```python
from build123d import *

# Parameters (mm, degrees)
SKETCH1_W           = 100
SKETCH1_H           = 275
BOSS_EXTRUDE1_DEPTH = 10
SKETCH2_W           = 60
SKETCH2_H           = 5
BOSS_EXTRUDE2_DEPTH = 5
SKETCH3_R           = 10
CUT_EXTRUDE1_DEPTH  = 152.348108677


with BuildPart() as part:
    # Sketch1 → Boss-Extrude1 (new body)
    with BuildSketch(Plane.XY):
        Rectangle(SKETCH1_W, SKETCH1_H)
    extrude(amount=BOSS_EXTRUDE1_DEPTH)

    # Sketch2 → Boss-Extrude2 (add)
    with BuildSketch(Plane(origin=(0, 137.5, 0), x_dir=(1, 0, 0), z_dir=(0, 1, 0))):
        with Locations((0, -5)):
            Rectangle(SKETCH2_W, SKETCH2_H)
    extrude(amount=BOSS_EXTRUDE2_DEPTH)

    # Sketch3 → Cut-Extrude1 (cut, through all)
    with BuildSketch(Plane.XY.offset(10)):
        with Locations((25, -117.5)):
            Circle(SKETCH3_R)
        with Locations(Location((-25, -117.5, 0), (0, 0, 180))):
            Circle(SKETCH3_R)
    extrude(amount=-CUT_EXTRUDE1_DEPTH, mode=Mode.SUBTRACT)


solid = part.part
```
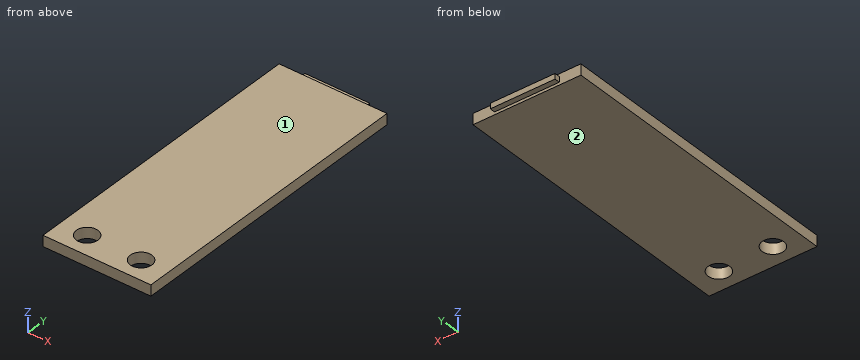
Read the model definition and answer for the solid it produces. Units are mm, in the model's axes. Face numbers are marked on the shaded views. Give positions to 0.01 mm unless a question says otherwise; leave off trailing zeros. Write each loop counter-clockwise with the first axis right and the second up, starting at its lowest first coordinate (ties: lowest second). Pieces come first, ordered by that corner, then holes. Notation, with made-up numbers: (66, -22.75) - (116, -22.75) arc R12 ccw to (116, -11.75) - close; hole circle Ø8 at (-35, -11.75). An arc over 180 degrees is marked (long way). Write item = value, one per line. Start each with the question number.
Item 1: Find section A-A (y = -117.5). Give the vertices of the cut face in (x, z).
Item 2: Find section C-C (z = 4.25). Give the vertices of the cut face in (x, y).
Item 3: The mould has two halves that part along Z. Classify the marked faces 1 and 2: +Z half, -Z half, draft (parallel to the pull), parting line (faces both ways), or undercut.
Item 4: Find section B-B (x = -25). Give the vertices of the cut face in (y, z), then the cut area to 4 significant figures.
Item 5: Find the intervals of material crossed by probe 1 along Y at (x, z) = (25, 6); probe 2 along Y at (x, z) = (-28.5, 8); probe 3 along X at (y, z) = (-109.5, 7), in increasing order. Write a range as [from, to].
Item 6: Each of these flat-tipped pins is pushed along its axis until it touches: P1, Ø4, axis at y = 140.5, z = 5, coming from the +X side; P2, Ø2.5, axis at y = 141, z = 4, coming from the -X side. Where does it stop, or does it pass through?
Response:
q1.outline = (-50, 0) - (-35, 0) - (-35, 10) - (-50, 10) - close; (-15, 0) - (15, 0) - (15, 10) - (-15, 10) - close; (35, 0) - (50, 0) - (50, 10) - (35, 10) - close
q2.outline = (-50, -137.5) - (50, -137.5) - (50, 137.5) - (30, 137.5) - (30, 142.5) - (-30, 142.5) - (-30, 137.5) - (-50, 137.5) - close; hole circle Ø20 at (-25, -117.5); hole circle Ø20 at (25, -117.5)
q3.face_1 = +Z half
q3.face_2 = -Z half
q4.outline = (-137.5, 0) - (-127.5, 0) - (-127.5, 10) - (-137.5, 10) - close; (-107.5, 0) - (137.5, 0) - (137.5, 2.5) - (142.5, 2.5) - (142.5, 7.5) - (137.5, 7.5) - (137.5, 10) - (-107.5, 10) - close
q4.area = 2,575 mm²
q5.probe_1 = [-137.5, -127.5], [-107.5, 142.5]
q5.probe_2 = [-137.5, -126.87], [-108.13, 137.5]
q5.probe_3 = [-50, -31], [-19, 19], [31, 50]
q6.P1 = 30
q6.P2 = -30
